Autodesk Inventor part; units mm, degrees
ref_plane "YZ Plane" through (0, 0, 0) normal (1, 0, 0) x (0, 1, 0)
ref_plane "XZ Plane" through (0, 0, 0) normal (0, 1, 0) x (-1, 0, 0)
ref_plane "XY Plane" through (0, 0, 0) normal (0, 0, 1) x (1, 0, 0)
sketch "Sketch1" plane through (0, 0, 0) normal (1, 0, 0) x (0, 1, 0)
  line L0 (0, 0) -> (381, 0)
  line L1 (381, 0) -> (381, -381)
  line L2 (381, -381) -> (0, -381)
  line L3 (0, -381) -> (0, 0)
  dimension "d0" = 381
  dimension "d1" = 381
extrude "Extrusion1" add sketch "Sketch1" along normal blind 12.7
sketch "Sketch2" plane through (0, 0, 0) normal (-1, 0, 0) x (0, 0, 1)
  line L0 (-355.6, 355.6) -> (-25.4, 355.6)
  line L1 (-25.4, 355.6) -> (-25.4, 25.4)
  line L2 (-25.4, 25.4) -> (-355.6, 25.4)
  line L3 (-355.6, 25.4) -> (-355.6, 355.6)
  line L4 (-381, 0) -> (-381, 381)
  line L5 (0, 381) -> (0, 0)
  line L6 (0, 0) -> (-381, 0)
  line L7 (-381, 381) -> (0, 381)
  dimension "d4" = 25.4
  dimension "d5" = 25.4
  dimension "d6" = 25.4
  dimension "d7" = 25.4
extrude "Extrusion2" add sketch "Sketch2" along normal blind 12.7 contours L0 L1 L2 L3
sketch "Sketch3" plane through (-12.7, 0, 0) normal (-1, 0, 0) x (0, 0, 1)
  line L0 (-330.2, 76.2) -> (-279.4, 76.2)
  line L1 (-279.4, 76.2) -> (-279.4, 50.8)
  line L2 (-279.4, 50.8) -> (-330.2, 50.8)
  line L3 (-330.2, 50.8) -> (-330.2, 76.2)
  line L4 (-355.6, 355.6) -> (-355.6, 25.4)
  line L5 (-355.6, 25.4) -> (-25.4, 25.4)
  point P0 (0, 0)
  dimension "d10" = 25.4
  dimension "d11" = 25.4
  dimension "d12" = 25.4
  dimension "d13" = 50.8
extrude "Extrusion3" add sketch "Sketch3" along normal blind 5.08
sketch "Sketch4" plane through (-12.7, 0, 0) normal (-1, 0, 0) x (0, 0, 1)
  line L0 (-101.6, 76.2) -> (-50.8, 76.2)
  line L1 (-50.8, 76.2) -> (-50.8, 50.8)
  line L2 (-50.8, 50.8) -> (-101.6, 50.8)
  line L3 (-101.6, 50.8) -> (-101.6, 76.2)
  line L4 (-25.4, 25.4) -> (-25.4, 355.6)
  line L5 (-355.6, 25.4) -> (-25.4, 25.4)
  point P0 (0, 0)
  dimension "d16" = 25.4
  dimension "d17" = 25.4
  dimension "d18" = 25.4
  dimension "d19" = 50.8
extrude "Extrusion4" add sketch "Sketch4" along normal blind 5.08
sketch "Sketch5" plane through (-17.78, 0, 0) normal (-1, 0, 0) x (0, 0, 1)
  line L0 (-317.5, 69.85) -> (-292.1, 69.85)
  line L1 (-292.1, 69.85) -> (-292.1, 57.15)
  line L2 (-292.1, 57.15) -> (-317.5, 57.15)
  line L3 (-317.5, 57.15) -> (-317.5, 69.85)
  line L4 (-279.4, 50.8) -> (-279.4, 76.2)
  line L5 (-330.2, 76.2) -> (-330.2, 50.8)
  line L6 (-279.4, 76.2) -> (-330.2, 76.2)
  line L7 (-330.2, 50.8) -> (-279.4, 50.8)
  point P0 (0, 0)
  dimension "d22" = 12.7
  dimension "d23" = 12.7
  dimension "d24" = 6.35
  dimension "d25" = 6.35
extrude "Extrusion5" cut sketch "Sketch5" against normal blind 5.08 contours L0 L1 L2 L3
sketch "Sketch6" plane through (-17.78, 0, 0) normal (-1, 0, 0) x (0, 0, 1)
  line L0 (-88.9, 69.85) -> (-63.5, 69.85)
  line L1 (-63.5, 69.85) -> (-63.5, 57.15)
  line L2 (-63.5, 57.15) -> (-88.9, 57.15)
  line L3 (-88.9, 57.15) -> (-88.9, 69.85)
  line L4 (-101.6, 76.2) -> (-101.6, 50.8)
  line L5 (-50.8, 50.8) -> (-50.8, 76.2)
  line L6 (-50.8, 76.2) -> (-101.6, 76.2)
  line L7 (-101.6, 50.8) -> (-50.8, 50.8)
  point P0 (0, 0)
  dimension "d28" = 12.7
  dimension "d29" = 12.7
  dimension "d30" = 6.35
  dimension "d31" = 6.35
extrude "Extrusion6" cut sketch "Sketch6" against normal blind 5.08 contours L0 L1 L2 L3
properties part number "front"
The model under review builds one solid part; all positions refer to its coordinate system, in mm. A direction names the side the tool comes from. Round coordinates to 2 decimals unless told otherwise and drop trailing zeros. Write each loop counter-clockwise with the first axis right and the second up, starting at its lowest first coordinate (ties: lowest second). Pieces come first, ordered by that corner, then holes.
(1) We need section D-D on z = -266. Give the boundary of the cut face in (x, y).
(2) Insertion check: pin 1 (2.5 mm diameter, centred on x = -14.5, z = -311.5, fed in from -Y); pin 2 (6.5 mm diameter, centred on y = 63, z = -74, fed in from -X); pin 3 (4 mm diameter, centred on x = -14, y = 60.5, fed in from +Z). Each pin has a flat end and moves straight along its axis. Give the tip position at first contact, or say it passes through.
(3) Machinability: for faces 1 (the flat face through (-12.7, 64, -305)), 2 (the flat face through (-6, 355.6, -193)), 3 (the flat face through (-6, 25.4, -188)), which of the approach directions +Z, -Z, +X, -X, +Y, -Y give a long, thin tool a straight path to every point of the face, cutting with its end or side? Answer none if there is none.
(4) We need section A-A on y = 119.5. Give the boundary of the cut face in (x, z).
(5) Wall thickness on L1, parallel to Y at x = -14, z = -298.5; L2, parallel to X at y = 147, z = -35; L3, parallel to Y at x = -12, z = -283: over which ranges is each line inside the solid? List them lowest first.
(6) We need section B-B on z = -304.5. Give the boundary of the cut face in (x, y).
(7) We need section C-C on x = -6. Give the boundary of the cut face in (y, z).
Findings below:
1. outline: (-12.7, 25.4) - (0, 25.4) - (0, 0) - (12.7, 0) - (12.7, 381) - (0, 381) - (0, 355.6) - (-12.7, 355.6) - close
2. pin 1: stops at y = 50.8
2. pin 2: stops at x = -12.7
2. pin 3: stops at z = -25.4
3. face 1: -X
3. face 2: +Z, -Z, -X, +Y
3. face 3: +Z, -Z, -X, -Y
4. outline: (-12.7, -355.6) - (0, -355.6) - (0, -381) - (12.7, -381) - (12.7, 0) - (0, 0) - (0, -25.4) - (-12.7, -25.4) - close
5. L1: y = 50.8 to 57.15, 69.85 to 76.2
5. L2: x = -12.7 to 12.7
5. L3: y = 25.4 to 355.6
6. outline: (-17.78, 50.8) - (-12.7, 50.8) - (-12.7, 25.4) - (0, 25.4) - (0, 0) - (12.7, 0) - (12.7, 381) - (0, 381) - (0, 355.6) - (-12.7, 355.6) - (-12.7, 76.2) - (-17.78, 76.2) - (-17.78, 69.85) - (-12.7, 69.85) - (-12.7, 57.15) - (-17.78, 57.15) - close
7. outline: (25.4, -355.6) - (355.6, -355.6) - (355.6, -25.4) - (25.4, -25.4) - close
